Geometry: see drawing. Coordinates: mm, zero at the bounding-box minimum. A direction names the side the tool comes from. Round coordinates to 2 decimals unless told otherwise and drop trailing zeros. Write each loop counter-clockwise with the first axis right and the second up, starting at its lowest first coordinate (ties: lowest second). Pieces come first, ordered by that corner, then holes. Notation, with made-up numbers: M 30.25,-27 L 68.25,-27 A4 ccw 68.25,-22 Z; hole C 45,25 d11. An arc over 180 degrees is marked long. Use one line per item in the form item = value. Start each with the question number.
Item 1: Ray query, probe 1 along Y at (x, z) = (25, 1.55); probe 2 along Z at (x, y) = (29, 30); probe 3 along Y at (x, z) = (25, 6.4) (3 decimals). Return the intervals inside material, ascending.
Item 2: Pin query (flat end, axial travel): pin 1 Ø1.5 at (x, y) = (37, 36) entering from -Z; pin 2 Ø7 at (x, y) = (25, 25) entering from -Z; pin 3 Ø4 at (y, z) = (39.5, 3.5) entering from -X; pin 4 Ø1 at (x, z) = (21.5, 4) entering from -Y. Return the tip coordinate at first contact, or that it passes through.
Item 3: Section query A-A (x = 25). Return loops of the section in (y, z) (3 decimals), and give its area (3 significant figures).
Item 4: Pull-direction query (X, two-part tool) for the marked faces 1, 2 and 3; classes: pulls with the +X half, pulls with the -X half, needs draft (parallel to the pull), parting line crosses it, or undercut.
Item 5: Section query B-B (z = 1.5). Return loops of the section in (x, y), and give its area (3 significant figures).
Item 6: Reachability of the marked faces 4 and 5 from +Z, -Z, +X, -X, +Y, -Y: full face, straight path, thin tool, end or side. Return the list, or none.
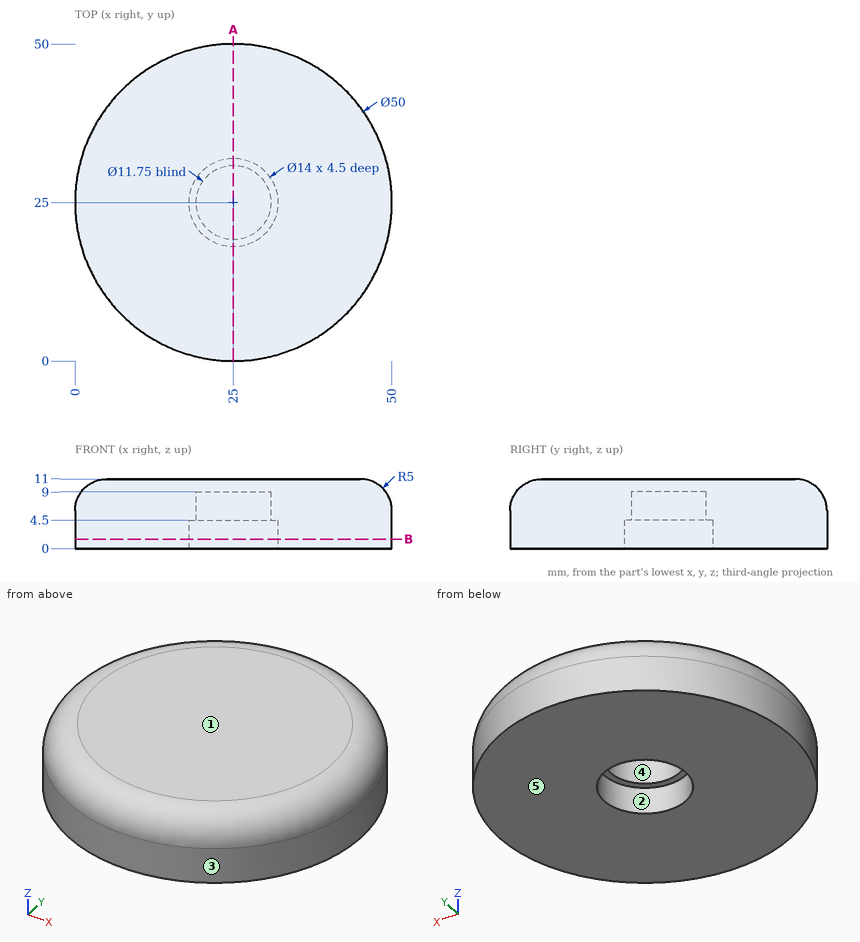
Working result:
q1.probe_1 = 0 to 18, 32 to 50
q1.probe_2 = 4.5 to 11
q1.probe_3 = 0.016 to 19.125, 30.875 to 49.984
q2.pin_1 = 0
q2.pin_2 = 9
q2.pin_3 = 3.35
q2.pin_4 = 0.18
q3.outline = M 0,0 L 18,0 L 18,4.5 L 19.125,4.5 L 19.125,9 L 30.875,9 L 30.875,4.5 L 32,4.5 L 32,0 L 50,0 L 50,6 A5 ccw 45,11 L 5,11 A5 ccw 0,6 Z
q3.area = 423 mm²
q4.face_1 = needs draft
q4.face_2 = undercut
q4.face_3 = parting line crosses it
q5.outline = C 25,25 d50; hole C 25,25 d14
q5.area = 1,810 mm²
q6.face_4 = -Z
q6.face_5 = -Z, +X, -X, +Y, -Y
